Autodesk Fusion 360 part; units mm, degrees
sketch "movingPlatform" plane through (0, 0, 0) normal (0, 0, 1) x (1, 0, 0)
  line L0 (-75, 59) -> (75, 59)
  line L1 (75, 59) -> (75, -59)
  line L2 (75, -59) -> (-75, -59)
  line L3 (-75, -59) -> (-75, 59)
  line L4 (-75, 59) -> (75, -59) construction
  line L5 (75, 59) -> (-75, -59) construction
  circle A0 centre (-60, -34) radius 6.65
  line L6 (0, 2.5) -> (0, 20)
  circle A1 centre (60, -34) radius 6.65
  circle A2 centre (0, 34) radius 6.4
  circle A3 centre (-46, -46) radius 1.588
  circle A4 centre (-15.5, -15.5) radius 1.588
  circle A5 centre (0, 0) radius 57 construction
  circle A6 centre (15.5, -15.5) radius 1.588
  circle A7 centre (15.5, 15.5) radius 1.588
  circle A8 centre (46, -46) radius 1.588
  circle A9 centre (-46, 46) radius 1.588
  circle A10 centre (46, 46) radius 1.588
  circle A11 centre (-15.5, 15.5) radius 1.588
  circle A12 centre (0, 0) radius 1.588
  dimension "d1" = 150
  dimension "d2" = 118
  dimension "d3" = 13.3
  dimension "d4" = 120
  dimension "d5" = 12.8
  dimension "d6" = 68
  dimension "d7" = 25
  dimension "d8" = 25
  dimension "d9" = 3.176
  dimension "d12" = 92
  dimension "d13" = 92
  dimension "d21" = 3.176
  dimension "d24" = 31
  dimension "d25" = 31
  dimension "d27" = 15.5
  dimension "d31" = 114
  dimension "d34" = 46
  dimension "d37" = 46
  dimension "d49" = 15.5
  dimension "d52" = 3.176
extrude "Extrude3" add sketch "movingPlatform" along normal blind 3.175
equation "d4 = 132.800 mm - 12.8 mm"
Geometry check sheet. Reference: the model listing, model coordinates, mm. Round coordinates to 2 decimals unless told otherwise and drop trailing zeros. Order: outer loops, then holes, each group sorted by start corner. A loop starts at its lowest first (then second) coordinate and runs counter-clockwise, first axis right, second up. Notation, with made-up numbers: M 27,63.25 L 45,63.25 A32 ccw 45,99.25 Z; hole C 25,54 d2. An arc over 180 degrees is marked long. Answer as CSV lines item,"result".
1) Sectioned sample at C-C on y = 46. Record the cut outline in (x, z) (3 decimals), and give its area (3 significant figures).
Entries:
outline,"M -75,0 L -47.588,0 L -47.588,3.175 L -75,3.175 Z; M -44.412,0 L 44.412,0 L 44.412,3.175 L -44.412,3.175 Z; M 47.588,0 L 75,0 L 75,3.175 L 47.588,3.175 Z"
area,"456 mm2"
2) Mould release check, pull along Y, two halves, no side actions. Record for faces 1 (the face through (1, -59, 2)), 2 (the face through (58.6, -27.5, 1.6)), 3 (the face through (-1, -12, 3.175)): +Y half, -Y half, draft (parallel to the pull), parting line (faces both ways), or undercut.
Entries:
face 1,"-Y half"
face 2,"undercut"
face 3,"draft"
3) Sectioned sample at A-A on x = -15.5. Record the cut outline in (y, z) (3 decimals), and give its area (3 significant figures).
Entries:
outline,"M -59,0 L -17.088,0 L -17.088,3.175 L -59,3.175 Z; M -13.912,0 L 13.912,0 L 13.912,3.175 L -13.912,3.175 Z; M 17.088,0 L 59,0 L 59,3.175 L 17.088,3.175 Z"
area,"354 mm2"
4) Gauge pin test, flat end, axial feed: pin 1 Ø8 at (x, y) = (-60, -34) entering from +Z. Record the tip position at first contact, or that the pin passes through.
Entries:
pin 1,"through"
5) Thickness scan on probe 1 along Y at (x, z) = (15.5, 2.2); probe 2 along Y at (x, z) = (60, 1.5); probe 3 along X at (y, z) = (45.5, 1.35). Record the ranges inside material, lowest first. Write a range as [from, to].
Entries:
probe 1,"[-59, -17.09], [-13.91, 13.91], [17.09, 59]"
probe 2,"[-59, -40.65], [-27.35, 59]"
probe 3,"[-75, -47.51], [-44.49, 44.49], [47.51, 75]"
6) Sectioned sample at B-B on x = 60. Record the cut outline in (y, z) (3 decimals).
Entries:
outline,"M -59,0 L -40.65,0 L -40.65,3.175 L -59,3.175 Z; M -27.35,0 L 59,0 L 59,3.175 L -27.35,3.175 Z"
7) Sectioned sample at D-D on z = 0.9. Give the number of separate pieces and of enclosed holes in the cut face, and give its area (3 significant figures).
Entries:
separate pieces,"1"
enclosed holes,"12"
area,"17,200 mm2"
